from build123d import *

# Parameters (mm, degrees)
BOSS_EXTRUDE1_DEPTH     = 19.05
SKETCH2_W               = 19.05
SKETCH2_H               = 6.35
CUT_EXTRUDE1_DEPTH      = 8.62
CUT_EXTRUDE1_DEPTH_BACK = 8.62
SKETCH3_R               = 3.81
CUT_EXTRUDE2_DEPTH      = 20.05
FILLET1_R               = 0.508


with BuildPart() as part:
    # Sketch1 → Boss-Extrude1 (new body)
    with BuildSketch(Plane.XY):
        with BuildLine():
            Line((0, 7.62), (-25.4, 7.62))
            Line((-25.4, 7.62), (-25.4, -7.62))
            Line((-25.4, -7.62), (0, -7.62))
            ThreePointArc((0, -7.62), (7.62, 0), (0, 7.62))
        make_face()
    extrude(amount=BOSS_EXTRUDE1_DEPTH)

    # Sketch2 → Cut-Extrude1 (cut, two sides)
    with BuildSketch(Plane(origin=(0, 0, 0), x_dir=(1, 0, 0), z_dir=(0, 1, 0))) as cut_extrude1_sk:
        with Locations((-1.905, -9.525)):
            Rectangle(SKETCH2_W, SKETCH2_H)
    extrude(amount=CUT_EXTRUDE1_DEPTH, mode=Mode.SUBTRACT)
    extrude(cut_extrude1_sk.sketch, amount=-CUT_EXTRUDE1_DEPTH_BACK, mode=Mode.SUBTRACT)

    # Sketch3 → Cut-Extrude2 (cut, through all)
    with BuildSketch(Plane.XY.offset(19.05)):
        Circle(SKETCH3_R)
    extrude(amount=-CUT_EXTRUDE2_DEPTH, mode=Mode.SUBTRACT)

    # Fillet1
    fillet1_edges = [part.edges().sort_by_distance(p)[0] for p in [
        (-12.7, -7.62, 19.05),
        (7.62, 0, 19.05),
        (-12.7, -7.62, 0),
        (-12.7, 7.62, 0),
        (7.62, 0, 0),
        (-12.7, 7.62, 19.05),
    ]]
    fillet(fillet1_edges, radius=FILLET1_R)


solid = part.part
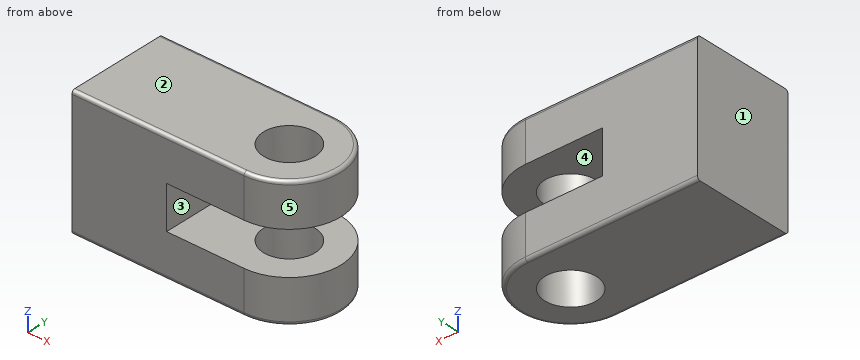
Geometry: final body of the model. Coordinates: model frame, mm. Face numbers are marked on the shaded views. A direction names the side the tool comes from. Coordinates: 2 decimals unless noted, no trailing zeros. Loops run counter-clockwise (first coordinate to the right, second up) from the corner with the lowest first, then second, coordinate; pieces in that order, holes last. Notation, with made-up numbers: M 14,-16.5 L 59,-16.5 A38 ccw 59,21.5 Z; hole C 37,57 d10. An arc over 180 degrees is marked long. One line per item, written item: value. Start each with the question number.
1) Cut plane A-A (y = 0). Return loops of the section in (x, z).
2) Cut plane C-C (z = 11.75). Return loops of the section in (x, y).
3) Material intervals for L1, parallel to Z at x = -5, y = 0; L2, parallel to Y at x = 0, z = 4.5; L3, parallel to X at y = 5.5, z = 9.5, sorted ascending. Write a range as from..to.
4) Pin query (flat end, axial travel): P1, Ø2, axis at y = -2.5, z = 9.5, coming from the +X side. Return the tip coordinate at first contact, or that it passes through.
5) Draft query along Z for the marked faces 1, 2 and 3. Return one class per face: released by +Z, released by -Z, zero draft, split by the parting line, or undercut.
6) Cut plane B-B (z = 15). Return loops of the section in (x, y).
7) Reachability of the marked faces 4 and 5 from +Z, -Z, +X, -X, +Y, -Y: full face, straight path, thin tool, end or side. Return the list, or none.
Evaluation:
1. outline: M -25.4,0 L -3.81,0 L -3.81,6.35 L -11.43,6.35 L -11.43,12.7 L -3.81,12.7 L -3.81,19.05 L -25.4,19.05 Z; M 3.81,0 L 7.11,0 A0.51 ccw 7.62,0.51 L 7.62,6.35 L 3.81,6.35 Z; M 3.81,12.7 L 7.62,12.7 L 7.62,18.54 A0.51 ccw 7.11,19.05 L 3.81,19.05 Z
2. outline: M -25.4,-7.62 L -11.43,-7.62 L -11.43,7.62 L -25.4,7.62 Z
3. L1: 0..6.35, 12.7..19.05
3. L2: -7.62..-3.81, 3.81..7.62
3. L3: -25.4..-11.43
4. P1: x = -11.43
5. face 1: zero draft
5. face 2: released by +Z
5. face 3: undercut
6. outline: M -25.4,-7.62 L 0,-7.62 A7.62 ccw 0,7.62 L -25.4,7.62 Z; hole C 0,0 d7.62
7. face 4: +X, +Y, -Y
7. face 5: +Z, -Z, +X
